```python
from build123d import *
from build123d import SkipClean  # not in build123d's __all__

# Parameters (mm, degrees)
F0_W      = 121.2
F0_H      = 121.2
F0_W_2    = 23
F0_H_2    = 23
F1_DEPTH  = 46
F0_R      = 8.75
F2_DEPTH  = 0.9
F3_W      = 121.2
F3_H      = 4
F4_DEPTH  = 2
F5_SIZE   = 1.99999
F7_DEPTH  = 2
F8_SIZE   = 1.99999
F9_W      = 121.2
F9_H      = 4
F10_DEPTH = 2
F11_SIZE  = 1.99999
F13_DEPTH = 2
F14_SIZE  = 1.99999
F15_W     = 1.5
F15_H     = 121.2
F16_DEPTH = 4


# Not quite as in the source:
# - a fillet or chamfer is up to 0.001 mm smaller than in the source, because OpenCascade refuses the exact size
# - a feature names something its author has since deleted; it is built from what else it names


with BuildPart() as f1:
    # F0 (on Top) → F1 (new body)
    with BuildSketch(Plane.XY):
        Rectangle(F0_W, F0_H)
        Polygon((-59.1, 35.3), (-59.1, 36.1), (-59.1, 59.1), (-36.1, 59.1), (-35.3, 59.1), (-12.3, 59.1), (-11.5, 59.1), (11.5, 59.1), (12.3, 59.1), (35.3, 59.1), (36.1, 59.1), (59.1, 59.1), (59.1, 36.1), (59.1, 35.3), (59.1, 12.3), (59.1, 11.5), (59.1, -11.5), (59.1, -12.3), (59.1, -35.3), (59.1, -36.1), (59.1, -59.1), (36.1, -59.1), (35.3, -59.1), (12.3, -59.1), (11.5, -59.1), (-11.5, -59.1), (-12.3, -59.1), (-35.3, -59.1), (-36.1, -59.1), (-59.1, -59.1), (-59.1, -36.1), (-59.1, -35.3), (-59.1, -12.3), (-59.1, -11.5), (-59.1, 11.5), (-59.1, 12.3), align=None, mode=Mode.SUBTRACT)
        Polygon((-36.1, 36.1), (-59.1, 36.1), (-59.1, 35.3), (-36.1, 35.3), (-36.1, 12.3), (-59.1, 12.3), (-59.1, 11.5), (-36.1, 11.5), (-36.1, -11.5), (-59.1, -11.5), (-59.1, -12.3), (-36.1, -12.3), (-36.1, -35.3), (-59.1, -35.3), (-59.1, -36.1), (-36.1, -36.1), (-36.1, -59.1), (-35.3, -59.1), (-35.3, -36.1), (-12.3, -36.1), (-12.3, -59.1), (-11.5, -59.1), (-11.5, -36.1), (11.5, -36.1), (11.5, -59.1), (12.3, -59.1), (12.3, -36.1), (35.3, -36.1), (35.3, -59.1), (36.1, -59.1), (36.1, -36.1), (59.1, -36.1), (59.1, -35.3), (36.1, -35.3), (36.1, -12.3), (59.1, -12.3), (59.1, -11.5), (36.1, -11.5), (36.1, 11.5), (59.1, 11.5), (59.1, 12.3), (36.1, 12.3), (36.1, 35.3), (59.1, 35.3), (59.1, 36.1), (36.1, 36.1), (36.1, 59.1), (35.3, 59.1), (35.3, 36.1), (12.3, 36.1), (12.3, 59.1), (11.5, 59.1), (11.5, 36.1), (-11.5, 36.1), (-11.5, 59.1), (-12.3, 59.1), (-12.3, 36.1), (-35.3, 36.1), (-35.3, 59.1), (-36.1, 59.1), align=None)
        with Locations((-23.8, -23.8)):
            Rectangle(F0_W_2, F0_H_2, mode=Mode.SUBTRACT)
        with Locations((0, -23.8)):
            Rectangle(F0_W_2, F0_H_2, mode=Mode.SUBTRACT)
        with Locations((-23.8, 0)):
            Rectangle(F0_W_2, F0_H_2, mode=Mode.SUBTRACT)
        Rectangle(F0_W_2, F0_H_2, mode=Mode.SUBTRACT)
        with Locations((23.8, -23.8)):
            Rectangle(F0_W_2, F0_H_2, mode=Mode.SUBTRACT)
        with Locations((23.8, 0)):
            Rectangle(F0_W_2, F0_H_2, mode=Mode.SUBTRACT)
        with Locations((-23.8, 23.8)):
            Rectangle(F0_W_2, F0_H_2, mode=Mode.SUBTRACT)
        with Locations((0, 23.8)):
            Rectangle(F0_W_2, F0_H_2, mode=Mode.SUBTRACT)
        with Locations((23.8, 23.8)):
            Rectangle(F0_W_2, F0_H_2, mode=Mode.SUBTRACT)
    extrude(amount=F1_DEPTH)

    # F0 (on Top) → F2 (join)
    with BuildSketch(Plane.XY):
        with Locations((-47.6, 47.6)):
            Rectangle(F0_W_2, F0_H_2)
        with Locations((-47.6, 47.6)):
            Circle(F0_R, mode=Mode.SUBTRACT)
        with Locations((-23.8, 47.6)):
            Rectangle(F0_W_2, F0_H_2)
        with Locations((-23.8, 47.6)):
            Circle(F0_R, mode=Mode.SUBTRACT)
        with Locations((0, 47.6)):
            Rectangle(F0_W_2, F0_H_2)
        with Locations((0, 47.6)):
            Circle(F0_R, mode=Mode.SUBTRACT)
        with Locations((23.8, 47.6)):
            Rectangle(F0_W_2, F0_H_2)
        with Locations((23.8, 47.6)):
            Circle(F0_R, mode=Mode.SUBTRACT)
        with Locations((47.6, 47.6)):
            Rectangle(F0_W_2, F0_H_2)
        with Locations((47.6, 47.6)):
            Circle(F0_R, mode=Mode.SUBTRACT)
        with Locations((47.6, 23.8)):
            Rectangle(F0_W_2, F0_H_2)
        with Locations((47.6, 23.8)):
            Circle(F0_R, mode=Mode.SUBTRACT)
        with Locations((23.8, 23.8)):
            Rectangle(F0_W_2, F0_H_2)
        with Locations((23.8, 23.8)):
            Circle(F0_R, mode=Mode.SUBTRACT)
        with Locations((0, 23.8)):
            Rectangle(F0_W_2, F0_H_2)
        with Locations((0, 23.8)):
            Circle(F0_R, mode=Mode.SUBTRACT)
        with Locations((-23.8, 23.8)):
            Rectangle(F0_W_2, F0_H_2)
        with Locations((-23.8, 23.8)):
            Circle(F0_R, mode=Mode.SUBTRACT)
        with Locations((-47.6, 23.8)):
            Rectangle(F0_W_2, F0_H_2)
        with Locations((-47.6, 23.8)):
            Circle(F0_R, mode=Mode.SUBTRACT)
        with Locations((-47.6, 0)):
            Rectangle(F0_W_2, F0_H_2)
        with Locations((-47.6, 0)):
            Circle(F0_R, mode=Mode.SUBTRACT)
        with Locations((-23.8, 0)):
            Rectangle(F0_W_2, F0_H_2)
        with Locations((-23.8, 0)):
            Circle(F0_R, mode=Mode.SUBTRACT)
        Rectangle(F0_W_2, F0_H_2)
        Circle(F0_R, mode=Mode.SUBTRACT)
        with Locations((23.8, 0)):
            Rectangle(F0_W_2, F0_H_2)
        with Locations((23.8, 0)):
            Circle(F0_R, mode=Mode.SUBTRACT)
        with Locations((47.6, 0)):
            Rectangle(F0_W_2, F0_H_2)
        with Locations((47.6, 0)):
            Circle(F0_R, mode=Mode.SUBTRACT)
        with Locations((47.6, -23.8)):
            Rectangle(F0_W_2, F0_H_2)
        with Locations((47.6, -23.8)):
            Circle(F0_R, mode=Mode.SUBTRACT)
        with Locations((23.8, -23.8)):
            Rectangle(F0_W_2, F0_H_2)
        with Locations((23.8, -23.8)):
            Circle(F0_R, mode=Mode.SUBTRACT)
        with Locations((0, -23.8)):
            Rectangle(F0_W_2, F0_H_2)
        with Locations((0, -23.8)):
            Circle(F0_R, mode=Mode.SUBTRACT)
        with Locations((-23.8, -23.8)):
            Rectangle(F0_W_2, F0_H_2)
        with Locations((-23.8, -23.8)):
            Circle(F0_R, mode=Mode.SUBTRACT)
        with Locations((-47.6, -23.8)):
            Rectangle(F0_W_2, F0_H_2)
        with Locations((-47.6, -23.8)):
            Circle(F0_R, mode=Mode.SUBTRACT)
        with Locations((-47.6, -47.6)):
            Rectangle(F0_W_2, F0_H_2)
        with Locations((-47.6, -47.6)):
            Circle(F0_R, mode=Mode.SUBTRACT)
        with Locations((-23.8, -47.6)):
            Rectangle(F0_W_2, F0_H_2)
        with Locations((-23.8, -47.6)):
            Circle(F0_R, mode=Mode.SUBTRACT)
        with Locations((0, -47.6)):
            Rectangle(F0_W_2, F0_H_2)
        with Locations((0, -47.6)):
            Circle(F0_R, mode=Mode.SUBTRACT)
        with Locations((23.8, -47.6)):
            Rectangle(F0_W_2, F0_H_2)
        with Locations((23.8, -47.6)):
            Circle(F0_R, mode=Mode.SUBTRACT)
        with Locations((47.6, -47.6)):
            Rectangle(F0_W_2, F0_H_2)
        with Locations((47.6, -47.6)):
            Circle(F0_R, mode=Mode.SUBTRACT)
    extrude(amount=F2_DEPTH)

    # F3 (on face) → F4 (join)
    with BuildSketch(Plane(origin=(-60.6, 0, 0), x_dir=(0, -1, 0), z_dir=(-1, 0, 0))):
        with Locations((0, 44)):
            Rectangle(F3_W, F3_H)
    extrude(amount=F4_DEPTH)

    # F5 (size 2 in the source; OpenCascade refuses exactly that, so slightly less here)
    f5_edges = [f1.edges().sort_by_distance(p)[0] for p in [
        (-62.6, 0, 42),
    ]]
    chamfer(f5_edges, length=F5_SIZE)

    # F6 (on face) → F7 (join)
    with BuildSketch(Plane.XZ.offset(60.6)):
        Polygon((-62.6, 44), (-60.6, 42), (60.6, 42), (60.6, 46), (-62.6, 46), align=None)
    with SkipClean():  # cleaning this boolean's faces spoils the solid; the shape is the same uncleaned
        extrude(amount=F7_DEPTH)

    # F8 (size 2 in the source; OpenCascade refuses exactly that, so slightly less here)
    f8_edges = [f1.edges().sort_by_distance(p)[0] for p in [
        (0, -62.6, 42),
    ]]
    chamfer(f8_edges, length=F8_SIZE)

    # F9 (on face) → F10 (join)
    with BuildSketch(Plane.YZ.offset(60.6)):
        with Locations((0, 44)):
            Rectangle(F9_W, F9_H)
        Polygon((-60.6, 42), (-60.6, 46), (-62.6, 46), (-62.6, 44), align=None)
    with SkipClean():  # cleaning this boolean's faces spoils the solid; the shape is the same uncleaned
        extrude(amount=F10_DEPTH)

    # F11 (size 2 in the source; OpenCascade refuses exactly that, so slightly less here)
    f11_edges = [f1.edges().sort_by_distance(p)[0] for p in [
        (62.6, 0, 42),
    ]]
    chamfer(f11_edges, length=F11_SIZE)

    # F12 (on face) → F13 (join)
    with BuildSketch(Plane(origin=(0, 60.6, 0), x_dir=(-1, 0, 0), z_dir=(0, 1, 0))):
        Polygon((62.6, 44), (62.6, 46), (-60.6, 46), (-60.6, 42), (60.6, 42), align=None)
        Polygon((-60.6, 42), (-60.6, 46), (-62.6, 46), (-62.6, 44), align=None)
    with SkipClean():  # cleaning this boolean's faces spoils the solid; the shape is the same uncleaned
        extrude(amount=F13_DEPTH)

    # F14 (size 2 in the source; OpenCascade refuses exactly that, so slightly less here)
    f14_edges = [f1.edges().sort_by_distance(p)[0] for p in [
        (0, 62.6, 42),
    ]]
    chamfer(f14_edges, length=F14_SIZE)

    # F15 (on face) → F16 (join)
    with BuildSketch(Plane.XY.offset(46)):
        Polygon((62.6, 62.6), (-62.6, 62.6), (-62.6, 60.6), (-61.1, 60.6), (-61.1, 61.1), (61.1, 61.1), (61.1, 60.6), (62.6, 60.6), align=None)
        with Locations((-61.85, 0)):
            Rectangle(F15_W, F15_H)
        Polygon((-61.1, -60.6), (-62.6, -60.6), (-62.6, -62.6), (60.6, -62.6), (60.6, -61.1), (-61.1, -61.1), align=None)
        Polygon((62.6, -62.6), (62.6, 60.6), (61.1, 60.6), (61.1, -61.1), (60.6, -61.1), (60.6, -62.6), align=None)
    with SkipClean():  # cleaning this boolean's faces spoils the solid; the shape is the same uncleaned
        extrude(amount=F16_DEPTH)


solid = f1.part
```
Build history of the part. All positions in model axes, mm. A direction names the side the tool comes from. Round coordinates to 2 decimals unless told otherwise and drop trailing zeros. Answer as CSV lines item,"result".
1. Wall check: probe 1 along Y at (x, z) = (25.5, 16); probe 2 along Y at (x, z) = (-47.6, 0.65). Give the ranges that are in metal, low to high. Write a range as [from, to].
Resolved:
probe 1,"y = [-60.6, -59.1], [-36.1, -35.3], [-12.3, -11.5], [11.5, 12.3], [35.3, 36.1], [59.1, 60.6]"
probe 2,"y = [-60.6, -56.35], [-38.85, -32.55], [-15.05, -8.75], [8.75, 15.05], [32.55, 38.85], [56.35, 60.6]"
2. 3-axis set-ups, long thin cutter, end or side, ignore diameter. For faces 1 (the cylindrical face through (-54.544, 18.476, 0.444)), 2 (the flat face through (16, 5, 0.9)): which of +Z, -Z, +X, -X, +Y, -Y reach the whole face in a straight line?
Resolved:
face 1,"+Z, -Z"
face 2,"+Z"
3. Cut at A-A on x = -47.6. Count the separate pieces of the cut face and the enclosed holes in it, then the cut area to 3 significant figures.
Resolved:
separate pieces,"6"
enclosed holes,"0"
area,"334 mm²"
4. Flat gauge pins, fed straight in: P1, Ø21, axis at y = 10, z = 21.5, coming from the -X side; P2, Ø3, axis at x = 48.5, z = 28, coming from the -Y side; P3, Ø6, axis at x = -12.5, z = 26, coming from the +Y side. Where does each tip first touch, or does it go through?
Resolved:
P1,"stops at x = -60.6"
P2,"stops at y = -60.6"
P3,"stops at y = 60.6"
